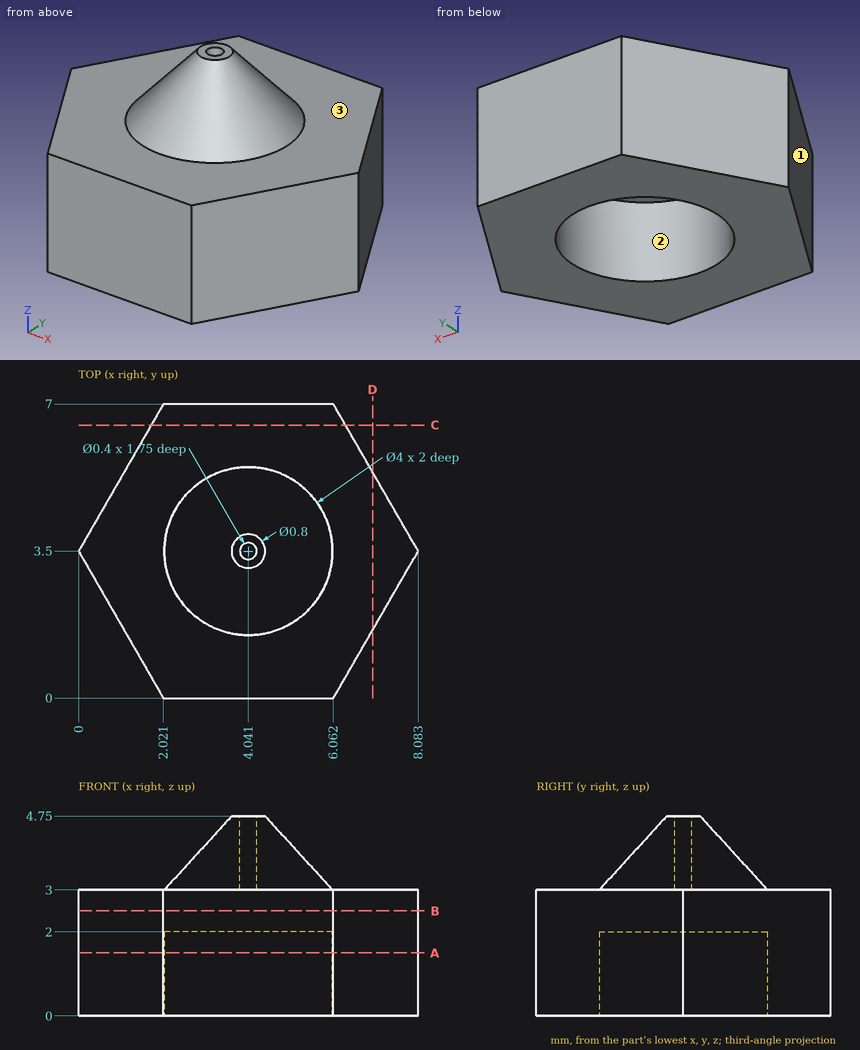
Input: dimensioned drawing with shaded views. Units: mm. Origin: part minimum x, y, z. A direction names the side the tool comes from. Coordinates: 2 decimals unless noted, no trailing zeros. Write each loop counter-clockwise with the first axis right and the second up, starting at its lowest first coordinate (ties: lowest second). Pieces come first, ordered by that corner, then holes. Notation, with made-up numbers: M -20.5,56.25 L 22.5,56.25 A21 ccw 22.5,62.25 Z; hole C 58.25,63 d10. An arc over 180 degrees is marked long. Answer as a JSON object with one key per item and string values. Group by question number.
(1) Set-up query: the marked faces 1, 2 and 3. Return all of +Z, -Z, +X, -X, +Y, -Y with unobstructed straight access to the full face (end or side cutting, diameter ignored); none if empty.
(2) Section B-B on z = 2.5. Output: boundary loops of the cut face in (x, y).
(3) Ray query, line 1 along Z through (x, y) = (5, 0.75); line 2 along Y through (x, z) = (5.25, 1.2) (1 decimal); line 3 along X through (y, z) = (3.5, 3.55) (1 decimal). Return the intervals inside material, ascending. Write a range as [from, to].
(4) Section C-C on y = 6.5. Output: boundary loops of the cut face in (x, z).
(5) Contact query for flat-ended pins moving along their axis: P1, Ø2, axis at x = 3.5, y = 3.5, coming from the -Z side; P2, Ø2, axis at y = 1, z = 2.5, coming from the +X side. Output: stop coordinate, or through.
(6) Section A-A on z = 1.5. Output: boundary loops of the cut face in (x, y).
(7) Section D-D on x = 7. Output: boundary loops of the cut face in (y, z) (1 decimal).
Result set:
{
 "1": {"face 1": "+Z, -Z, -X, -Y", "face 2": "-Z", "face 3": "+Z"},
 "2": {"outline": "M 0,3.5 L 2.02,0 L 6.06,0 L 8.08,3.5 L 6.06,7 L 2.02,7 Z"},
 "3": {"line 1": "z = [0, 3]", "line 2": "y = [0, 1.9], [5.1, 7]", "line 3": "x = [2.5, 3.8], [4.2, 5.5]"},
 "4": {"outline": "M 1.73,0 L 6.35,0 L 6.35,3 L 1.73,3 Z"},
 "5": {"P1": "stops at z = 2", "P2": "stops at x = 7.22"},
 "6": {"outline": "M 0,3.5 L 2.02,0 L 6.06,0 L 8.08,3.5 L 6.06,7 L 2.02,7 Z; hole C 4.04,3.5 d4"},
 "7": {"outline": "M 1.6,0 L 5.4,0 L 5.4,3 L 1.6,3 Z"}
}
